Study the drawing (mm; zero at the part's minimum x, y, z) and answer. A direction names the side the tool comes from. Round coordinates to 2 decimals unless told otherwise and drop trailing zeros. Order: outer loops, then holes, each group sorted by start corner. A loop starts at its lowest first (then second) coordinate and runs counter-clockwise, first axis right, second up. Notation, with made-up numbers: (-15, -11.5) -> (30, -11.5) arc R29 cw to (30, 21.5) -> close; hole circle Ø8 at (52.5, 12.25). An arc over 180 degrees is marked (long way). Answer in a Markdown table with one row per item. Add a question column.
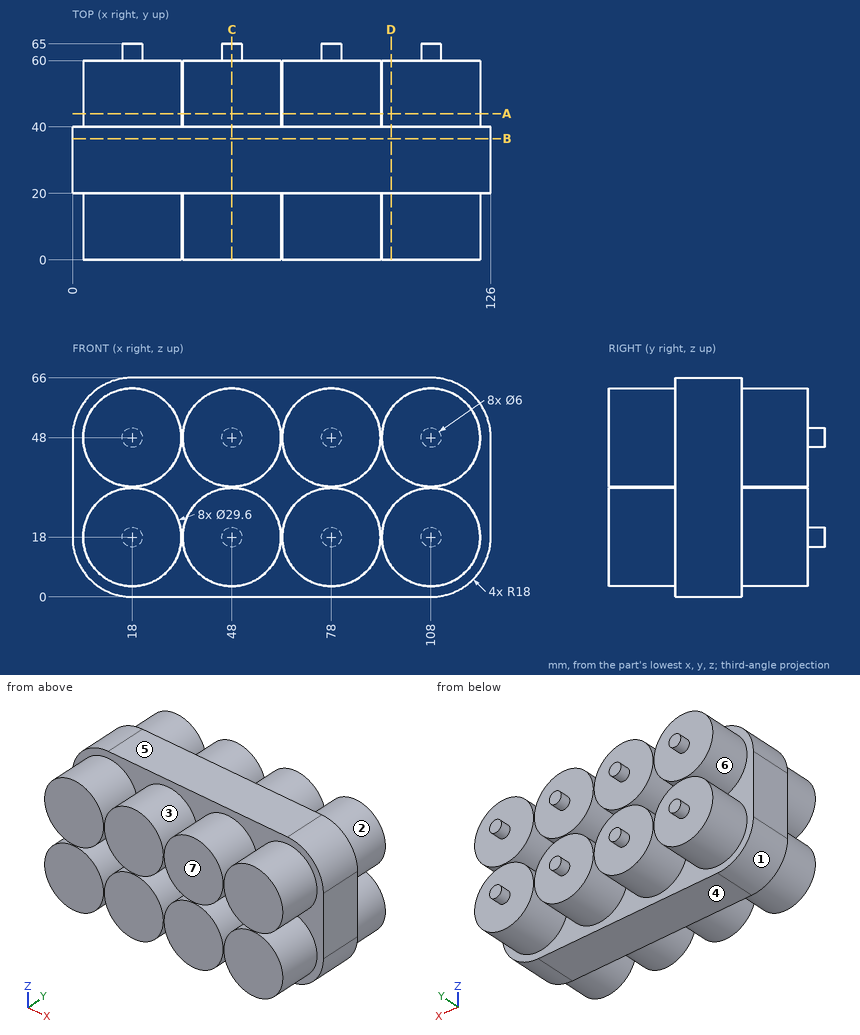
Item 1: Find the intervals of material crossed by probe 1 along X at (y, z) = (58.5, 48.5); probe 2 along Z at (x, y) = (18, 9); probe 3 along X at (y, z) = (59, 61.5), in increasing order. Write a range as [from, to].
Item 2: The part is cut by section A-A, the plane y = 44. Give the vertices of the cut face in (x, z), and give its area (3 significant figures).
Item 3: A tool of negligible diameter and unlimited length cuts with its end or side. For the marked faces 1, 2 and 3, from which of +Z, -Z, +X, -X, +Y, -Y can it reach the whole face along a straight path? Write none if from no direction.
Item 4: For a pull along Z with two mould halves and no side action, classify the marked faces 4, 5, 6 and 7 as released by +Z, released by -Z, zero draft, split by the parting line, or undercut.
Item 5: Flat-ended cylindrical pins translate along their axes: P1, Ø6, axis at x = 40, z = 41, coming from the +Y side; P2, Ø1.5, axis at x = 67.5, z = 36, coming from the +Y side; P3, Ø3, axis at x = 68, y = 11.5, coming from the -Z side. Find the tip coordinate at first contact, or state that the pin passes through.
Item 6: The part is cut by section C-C, the plane x = 48. Give the vertices of the cut face in (y, z).
Item 7: The part is cut by section D-D, the plane x = 96. Give the vertices of the cut face in (y, z).
Item 8: The part is cut by section B-B, the plane y = 36.5. Give the vertices of the cut face in (x, z).
Resolved:
| question | item | result |
|---|---|---|
| 1 | probe 1 | [3.21, 32.79], [33.21, 62.79], [63.21, 92.79], [93.21, 122.79] |
| 1 | probe 2 | [3.2, 32.8], [33.2, 62.8] |
| 1 | probe 3 | [11.93, 24.07], [41.93, 54.07], [71.93, 84.07], [101.93, 114.07] |
| 2 | outline | circle Ø29.6 at (18, 18); circle Ø29.6 at (18, 48); circle Ø29.6 at (48, 18); circle Ø29.6 at (48, 48); circle Ø29.6 at (78, 18); circle Ø29.6 at (78, 48); circle Ø29.6 at (108, 18); circle Ø29.6 at (108, 48) |
| 2 | area | 5,510 mm2 |
| 3 | face 1 | -Z, -X, +Y, -Y |
| 3 | face 2 | +Y |
| 3 | face 3 | -Y |
| 4 | face 4 | released by -Z |
| 4 | face 5 | released by +Z |
| 4 | face 6 | undercut |
| 4 | face 7 | zero draft |
| 5 | P1 | y = 60 |
| 5 | P2 | y = 40 |
| 5 | P3 | z = 5.88 |
| 6 | outline | (0, 3.2) -> (20, 3.2) -> (20, 0) -> (40, 0) -> (40, 3.2) -> (60, 3.2) -> (60, 15) -> (65, 15) -> (65, 21) -> (60, 21) -> (60, 32.8) -> (40, 32.8) -> (40, 33.2) -> (60, 33.2) -> (60, 45) -> (65, 45) -> (65, 51) -> (60, 51) -> (60, 62.8) -> (40, 62.8) -> (40, 66) -> (20, 66) -> (20, 62.8) -> (0, 62.8) -> (0, 33.2) -> (20, 33.2) -> (20, 32.8) -> (0, 32.8) -> close |
| 7 | outline | (0, 9.34) -> (20, 9.34) -> (20, 0) -> (40, 0) -> (40, 9.34) -> (60, 9.34) -> (60, 26.66) -> (40, 26.66) -> (40, 39.34) -> (60, 39.34) -> (60, 56.66) -> (40, 56.66) -> (40, 66) -> (20, 66) -> (20, 56.66) -> (0, 56.66) -> (0, 39.34) -> (20, 39.34) -> (20, 26.66) -> (0, 26.66) -> close |
| 8 | outline | (0, 18) arc R18 ccw to (18, 0) -> (108, 0) arc R18 ccw to (126, 18) -> (126, 48) arc R18 ccw to (108, 66) -> (18, 66) arc R18 ccw to (0, 48) -> close |
